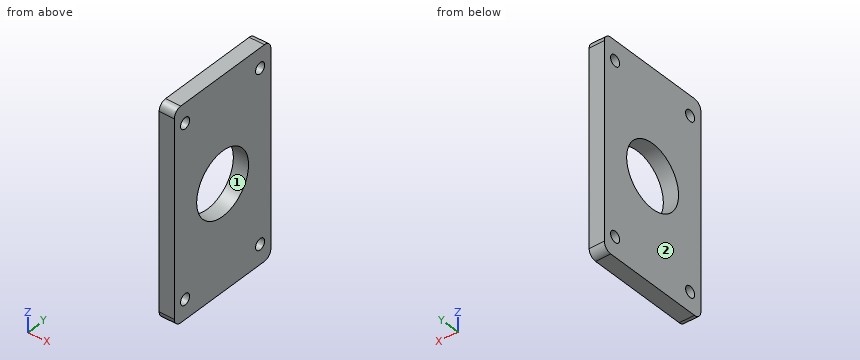
```python
from build123d import *

# Parameters (mm, degrees)
SKETCH_1_W      = 80
SKETCH_1_H      = 45
SKETCH_1_R      = 12.1
SKETCH_1_R_2    = 2.1
EXTRUDE_1_DEPTH = 5.8
FILLET_1_R      = 3


with BuildPart() as part:
    # ｽｹｯﾁ1 → ﾎﾞｽ - 押し出し1 (new body)
    with BuildSketch(Plane(origin=(0, 0, 0), x_dir=(0, 0, -1), z_dir=(1, 0, 0))):
        Rectangle(SKETCH_1_W, SKETCH_1_H)
        Circle(SKETCH_1_R, mode=Mode.SUBTRACT)
        with Locations((32.5, 17.5)):
            Circle(SKETCH_1_R_2, mode=Mode.SUBTRACT)
        with Locations(Location((32.5, -17.5, 0), (0, 0, 180))):
            Circle(SKETCH_1_R_2, mode=Mode.SUBTRACT)
        with Locations(Location((-32.5, 17.5, 0), (0, 0, 180))):
            Circle(SKETCH_1_R_2, mode=Mode.SUBTRACT)
        with Locations((-32.5, -17.5)):
            Circle(SKETCH_1_R_2, mode=Mode.SUBTRACT)
    extrude(amount=EXTRUDE_1_DEPTH)

    # ﾌｨﾚｯﾄ1
    fillet_1_edges = [part.edges().sort_by_distance(p)[0] for p in [
        (2.9, -22.5, -40),
        (2.9, -22.5, 40),
        (2.9, 22.5, 40),
        (2.9, 22.5, -40),
    ]]
    fillet(fillet_1_edges, radius=FILLET_1_R)


solid = part.part
```
Read the model definition and answer for the solid it produces. Units are mm, in the model's axes. Face numbers are marked on the shaded views. Give positions to 0.01 mm unless a question says otherwise; leave off trailing zeros. Write each loop counter-clockwise with the first axis right and the second up, starting at its lowest first coordinate (ties: lowest second). Pieces come first, ordered by that corner, then holes. Notation, with made-up numbers: (57.5, 43) - (98.5, 43) arc R29 cw to (98.5, 75) - close; hole circle Ø3 at (-38.75, 51). An arc over 180 degrees is marked (long way). Write item = value, one per line. Start each with the question number.
Item 1: Find the intervals of material crossed by probe 1 along Y at (x, z) = (2.45, 32.5); probe 2 along Z at (x, y) = (4.9, -18); probe 3 along Y at (x, z) = (3.7, 5), in increasing order. Write a range as [from, to].
Item 2: Find section B-B (y = 17.5). Give the vertices of the cut face in (x, z).
Item 3: Find section C-C (x = 4.2). Give the vertices of the cut face in (y, z), then the cut area to 3 significant figures.
Item 4: Each of these flat-tipped pins is pushed along its axis until it touches: P1, Ø5.5, axis at y = -17.5, z = -32.5, coming from the -X side; P2, Ø2.5, axis at y = -17.5, z = 32.5, coming from the +X side. Where does it stop, or does it pass through?
Item 5: The mould has two halves that part along Y. Classify the marked faces 1 and 2: +Y half, -Y half, draft (parallel to the pull), parting line (faces both ways), or undercut.
Item 6: Find section A-A (z = 32.5). Give the vertices of the cut face in (x, y), then the cut area to 3 significant figures.
Item 7: Find section D-D (z = 2). Give the vertices of the cut face in (x, y).
Response:
q1.probe_1 = [-22.5, -19.6], [-15.4, 15.4], [19.6, 22.5]
q1.probe_2 = [-40, -34.54], [-30.46, 30.46], [34.54, 40]
q1.probe_3 = [-22.5, -11.02], [11.02, 22.5]
q2.outline = (0, -40) - (5.8, -40) - (5.8, -34.6) - (0, -34.6) - close; (0, -30.4) - (5.8, -30.4) - (5.8, 30.4) - (0, 30.4) - close; (0, 34.6) - (5.8, 34.6) - (5.8, 40) - (0, 40) - close
q3.outline = (-22.5, -37) arc R3 ccw to (-19.5, -40) - (19.5, -40) arc R3 ccw to (22.5, -37) - (22.5, 37) arc R3 ccw to (19.5, 40) - (-19.5, 40) arc R3 ccw to (-22.5, 37) - close; hole circle Ø4.2 at (-17.5, -32.5); hole circle Ø4.2 at (-17.5, 32.5); hole circle Ø24.2 at (0, 0); hole circle Ø4.2 at (17.5, -32.5); hole circle Ø4.2 at (17.5, 32.5)
q3.area = 3,080 mm²
q4.P1 = 0
q4.P2 = through
q5.face_1 = undercut
q5.face_2 = draft
q6.outline = (0, -22.5) - (5.8, -22.5) - (5.8, -19.6) - (0, -19.6) - close; (0, -15.4) - (5.8, -15.4) - (5.8, 15.4) - (0, 15.4) - close; (0, 19.6) - (5.8, 19.6) - (5.8, 22.5) - (0, 22.5) - close
q6.area = 212 mm²
q7.outline = (0, -22.5) - (5.8, -22.5) - (5.8, -11.93) - (0, -11.93) - close; (0, 11.93) - (5.8, 11.93) - (5.8, 22.5) - (0, 22.5) - close
